Here's the drawing with two shaded views (mm, measured from the low corner). I have some questions. A direction names the side the tool comes from. Give positions to 0.01 mm unless a question says otherwise; leave off trailing zeros. Write each loop counter-clockwise with the first axis right and the second up, starting at its lowest first coordinate (ties: lowest second). Pieces come first, ordered by that corner, then holes. Notation, with made-up numbers: (46.5, 57.5) - (65.5, 57.5) arc R13 cw to (65.5, 67.5) - close; hole circle Ø5 at (45, -38.75). An arc over 180 degrees is marked (long way). Answer as CSV lines item,"result". Start each with the question number.
Q1. Imagine slicing it at B-B on x = 7.5. List the corners of the cut face in (y, z) for me, and give its area (3 significant figures).
Q2. Will these pins go through, and if not, where does the flat tip stop? pin 1 Ø1.5 at (y, z) = (5, 23) entering from -X; pin 2 Ø2 at (y, z) = (9, 13) entering from +X; pin 3 Ø1.5 at (x, y) = (25, 5) entering from -Z.
Q3. If I drill on line 1 along Z through (x, y) = (7.8, 17.4); line 2 along X through (y, z) = (18.5, 17.5); line 3 along Z through (x, y) = (28.5, 4), over which ranges is the centre line in solid material (lowest first)?
Q4. Imagine slicing it at D-D on z = 6. List the corners of the cut face in (x, y) for me.
Q5. On a 3-axis mill with a long thin cutter (end or side, diameter ignored), from which of +Z, -Z, +X, -X, +Y, -Y can I reach the whole of each face in a straight line? I mean the marked faces 1, 2 and 3. Say none if no direction works.
Q6. Imagine slicing it at A-A on y = 17.4. List the corners of the cut face in (x, z) for me.
Q7. Imagine slicing it at C-C on y = 20. List the corners of the cut face in (x, z) for me.
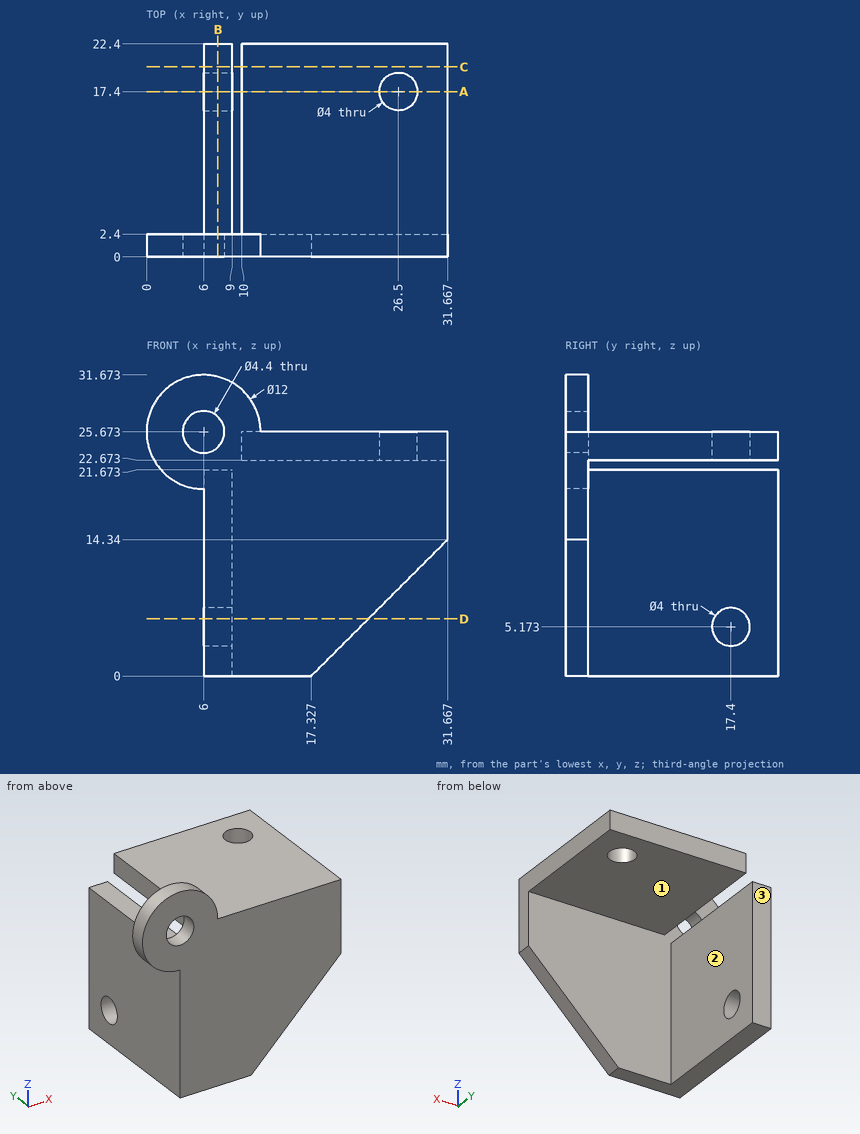
Conclusion:
1,outline,"(0, 0) - (22.4, 0) - (22.4, 21.67) - (2.4, 21.67) - (2.4, 24.06) - (0, 24.06) - close; (0, 27.28) - (2.4, 27.28) - (2.4, 31.48) - (0, 31.48) - close; hole circle Ø4 at (17.4, 5.17)"
1,area,"489 mm^2"
2,pin 1,"x = 10"
2,pin 2,"x = 9"
2,pin 3,"z = 22.67"
3,line 1,"0 to 3.17, 7.17 to 21.67"
3,line 2,"6 to 9"
3,line 3,"22.67 to 25.67"
4,outline,"(6, 0) - (23.33, 0) - (23.33, 2.4) - (9, 2.4) - (9, 15.58) - (6, 15.58) - close; (6, 19.22) - (9, 19.22) - (9, 22.4) - (6, 22.4) - close"
5,face 1,"-Z, +X, -X, +Y"
5,face 2,"+Z, -Z, +X, +Y"
5,face 3,"+Z, -Z, +X, -X, +Y"
6,outline,"(6, 0) - (9, 0) - (9, 3.17) - (6, 3.17) - close; (6, 7.17) - (9, 7.17) - (9, 21.67) - (6, 21.67) - close; (10, 22.67) - (24.5, 22.67) - (24.5, 25.67) - (10, 25.67) - close; (28.5, 22.67) - (31.67, 22.67) - (31.67, 25.67) - (28.5, 25.67) - close"
7,outline,"(6, 0) - (9, 0) - (9, 21.67) - (6, 21.67) - close; (10, 22.67) - (31.67, 22.67) - (31.67, 25.67) - (10, 25.67) - close"
